Here's how the part is built. I have some questions about the finished solid (model axes, mm). Face numbers are marked on the shaded views. A direction names the side the tool comes from. Round coordinates to 2 decimals unless told otherwise and drop trailing zeros. Write each loop counter-clockwise with the first axis right and the second up, starting at its lowest first coordinate (ties: lowest second). Pieces come first, ordered by that corner, then holes. Notation, with made-up numbers: M 49.5,-38 L 101.5,-38 A23 cw 101.5,-4 Z; hole C 20,-19.5 d6. An arc over 180 degrees is marked long. Write item = value, one per line. Start each with the question number.
(1) I need wall thicknesses on line 1 along X through (y, z) = (-0.25, -2.5); line 2 along X through (y, z) = (-1.5, 2.25); line 3 along Y through (x, z) = (-2.5, 2). Which ranges of each line are inside material? Lowest first, please.
(2) On a 3-axis mill with a long thin cutter (end or side, diameter ignored), from which of +Z, -Z, +X, -X, +Y, -Y can I reach the whole of each face in a straight line? I mean the marked faces 1, 2 and 3. Say none if no direction works.
(3) Will these pins go through, and if not, where does the flat tip stop? pin 1 Ø4 at (x, y) = (5, 1) entering from +Z; pin 2 Ø1.5 at (y, z) = (3, 1) entering from +X; pin 3 Ø1 at (x, z) = (5.5, 0) entering from +Y.
(4) I want a section at A-A (y = 0). List the corners of the cut face in (x, z) for me.
(5) I want a section at C-C (x = 5.25). List the corners of the cut face in (y, z) for me, and give its area (3 significant figures).
(6) I want a section at B-B (x = -1.25). List the corners of the cut face in (y, z) for me, and give its area (3 significant figures).
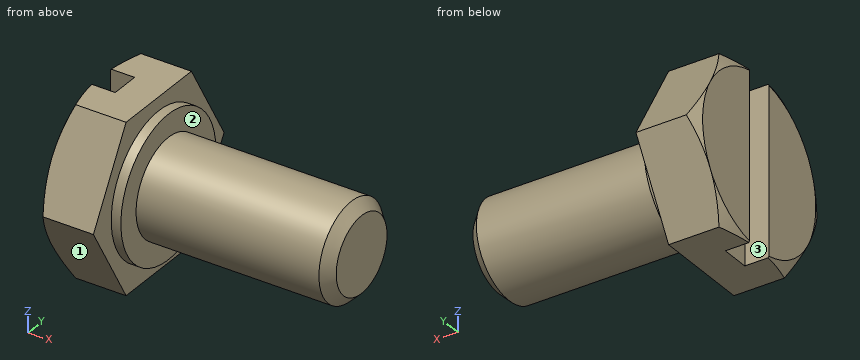
Autodesk Inventor part; units mm, degrees
ref_plane "Work Plane1" through (60, 0, 0) normal (0, 0, 1) x (1, 0, 0)
ref_plane "YZ Plane" through (0, 0, 0) normal (1, 0, 0) x (0, 1, 0)
ref_plane "XZ Plane" through (0, 0, 0) normal (0, 1, 0) x (-1, 0, 0)
sketch "Sketch1" plane through (0, 0, 0) normal (0, 0, 1) x (1, 0, 0)
  line L0 (0, 2.94) -> (0, 2)
  line L1 (0, 2) -> (8, 2)
  line L2 (8, 2) -> (8, 0)
  line L3 (8, 0) -> (-0.4001, 0)
  line L4 (-2.0801, 0) -> (9.68, 0)
  line L5 (-0.4001, 0) -> (-0.4001, 2.94)
  line L6 (-0.4001, 2.94) -> (0, 2.94)
  line L7 (0, -0.588) -> (0, 3.528)
  dimension "d0" = 8
  dimension "d1" = 4
  dimension "d8" = 0.4001
  dimension "d9" = 5.88
revolve "Body" add sketch "Sketch1" angle 360 about axis through (8, 0, 0) along (-1, 0, 0)
sketch "Sketch2" plane through (-0.4001, 0, 0) normal (-1, 0, 0) x (0, 0, 1)
  line L0 (0, 4.0415) -> (3.5, 2.0207)
  line L1 (3.5, 2.0207) -> (3.5, -2.0207)
  line L2 (3.5, -2.0207) -> (0, -4.0415)
  line L3 (0, -4.0415) -> (-3.5, -2.0207)
  line L4 (-3.5, -2.0207) -> (-3.5, 2.0207)
  line L5 (-3.5, 2.0207) -> (0, 4.0415)
  point P0 (0, 0)
  point P1 (0, 0)
  dimension "d10" = 7
extrude "Head" add sketch "Sketch2" along normal blind 2.4
sketch "Sketch3" plane through (0, 0, 0) normal (0, 0, 1) x (1, 0, 0)
  line L0 (-2.8001, 0.6) -> (-1.8001, 0.6)
  line L1 (-1.8001, 0.6) -> (-1.8001, -0.6)
  line L2 (-1.8001, -0.6) -> (-2.8001, -0.6)
  line L3 (-2.8001, -0.6) -> (-2.8001, 0.6)
  line L4 (-1.8001, 0) -> (-2.8001, 0) construction
  line L5 (-3.0001, 0) -> (-1.6001, 0)
  line L6 (-2.8001, 2.0207) -> (-2.8001, -2.0207)
  dimension "d11" = 1.2
  dimension "d13" = 1
extrude "Slot" cut sketch "Sketch3" along normal through all both and the other way through all
sketch "Sketch4" plane through (0, 0, 0) normal (0, 0, 1) x (1, 0, 0)
  line L0 (-2.8001, 3.5) -> (-2.8001, 4.0415)
  line L1 (-2.8001, 4.0415) -> (-2.4875, 4.0415)
  line L2 (-2.4875, 4.0415) -> (-2.8001, 3.5)
  line L3 (-2.4875, 4.0415) -> (-2.8001, 4.0415)
  line L4 (-2.8001, 4.0415) -> (-2.8001, 3.5)
  line L5 (-2.8001, 4.0415) -> (-2.8001, 2.0207)
  line L6 (-3.2801, 0) -> (0.0799, 0)
  line L7 (-0.4001, 4.0415) -> (-2.8001, 4.0415)
  dimension "d4" = 30
  dimension "d17" = 7
revolve "Chamfer1" cut sketch "Sketch4" angle 360 about axis through (-10, 0, 0) along (1, 0, 0)
thread "Thread"
chamfer "Chamfer2" distance 0.4294 distance2 0.4295 1 edges at (8, -2, 0) measured on face at (8, 0.6473, -0.1595)
ref_plane "Work Plane1" through (60, 0, 0) normal (0, 0, 1) x (1, 0, 0)
equation "\"d0\" = NLG"
equation "\"d1\" = GD"
equation "\"d9\" = SD2"
equation "\"d10\" = SW"
equation "\"d2\" = KOH - SD"
equation "\"d11\" = SBR"
equation "\"d13\" = STI"
equation "\"d4\" = ANG1"
equation "\"d17\" = SW0"
equation "\"d15\" = GEL"
equation "\"d5\" = -0.5 * SPD + 0.5 * GD"
equation "\"NLG\" = 8"
equation "\"GD\" = NND"
equation "\"KOH\" = 2.8"
equation "\"GEL\" = 7.3"
equation "\"SW\" = 7"
equation "\"SW0\" = SW"
equation "\"SPD\" = NND - 1.2269 * PTC"
equation "\"SD2\" = SDH"
equation "\"SD\" = WFT"
equation "\"ANG1\" = 30deg"
equation "\"GUL\" = 0.61345 * PTC"
equation "\"STI\" = 1"
equation "\"SBR\" = 1.2"
equation "\"RR\" = 0.2"
equation "\"GAL\" = 0.61345 * PTC"
equation "\"BDM\" = NND"
equation "\"WFT\" = 0.4"
equation "\"FAWI\" = 45deg"
equation "\"PTC\" = 0.7"
equation "\"THREADDIA\" = 4"
equation "\"E0\" = 1.155 * SW"
equation "\"TOA\" = 30deg"
equation "\"NND\" = 4"
equation "\"GD1\" = THREADDIA - 1.2269 * PTC"
equation "\"SDH\" = 5.88"
properties part number "Bolt GB/T 29.1 M4 x 8" material "Steel, Mild"
Returned:
q1.line_1 = -1.8 to 0
q1.line_2 = -2.8 to 0
q1.line_3 = -2.89 to -0.6, 0.6 to 2.89
q2.face_1 = -Z, +X, -X, -Y
q2.face_2 = +X
q2.face_3 = +Z, -Z, -X
q3.pin_1 = 2
q3.pin_2 = 0
q3.pin_3 = 2
q4.outline = M -1.8,-3.5 L -0.4,-3.5 L -0.4,-2.94 L 0,-2.94 L 0,-2 L 7.57,-2 L 8,-1.57 L 8,1.57 L 7.57,2 L 0,2 L 0,2.94 L -0.4,2.94 L -0.4,3.5 L -1.8,3.5 Z
q5.outline = C 0,0 d4
q5.area = 12.6 mm²
q6.outline = M -4.04,0 L -2.02,-3.5 L 2.02,-3.5 L 4.04,0 L 2.02,3.5 L -2.02,3.5 Z
q6.area = 42.4 mm²
